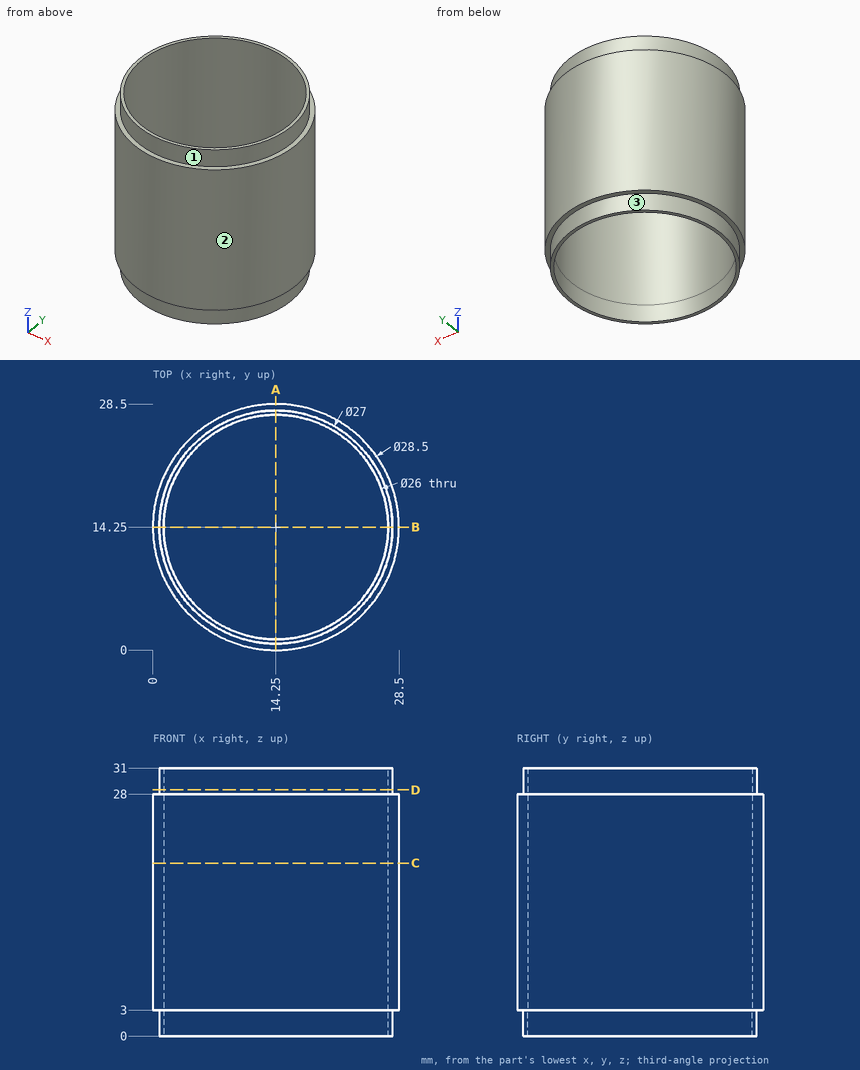
Design review of the part shown in the three views and the two pictorial views. Dimensions are in mm from the part's minimum x, y and z. A direction names the side the tool comes from. Round coordinates to 2 decimals unless told otherwise and drop trailing zeros. Order: outer loops, then holes, each group sorted by start corner. A loop starts at its lowest first (then second) coordinate and runs counter-clockwise, first axis right, second up. Notation, with made-up numbers: (-33.5, 32.25) - (-15.5, 32.25) arc R25 cw to (-15.5, 59.25) - close; hole circle Ø7 at (-40, 89). An arc over 180 degrees is marked (long way). Answer in a Markdown table with one row per item.
(1) Take a section at A-A on x = 14.25. Write out the cut boundary in (y, z).
Result set:
| item | result |
|---|---|
| outline | (0, 3) - (0.75, 3) - (0.75, 0) - (1.25, 0) - (1.25, 31) - (0.75, 31) - (0.75, 28) - (0, 28) - close; (27.25, 0) - (27.75, 0) - (27.75, 3) - (28.5, 3) - (28.5, 28) - (27.75, 28) - (27.75, 31) - (27.25, 31) - close |
(2) Take a section at D-D on z = 28.5. Write out the cut boundary in (x, y).
Result set:
| item | result |
|---|---|
| outline | circle Ø27 at (14.25, 14.25); hole circle Ø26 at (14.25, 14.25) |
(3) Clearance check with flat-ended pins moving along their axes: P1, Ø4, axis at x = 24.5, y = 3.5, coming from the -Z side; P2, Ø8, axis at x = 20.5, z = 26, coming from the +Y side; P3, Ø12, axis at y = 5, z = 16.5, coming from the +X side; P4, Ø8, axis at x = 7, y = 12.5, coming from the -Z side. State where each tip first meets the part, or that it passes through.
Result set:
| item | result |
|---|---|
| P1 | stops at z = 0 |
| P2 | stops at y = 28.32 |
| P3 | stops at x = 28.12 |
| P4 | passes through |
(4) Machinability: for the marked faces 1, 2 and 3, which of the approach directions +Z, -Z, +X, -X, +Y, -Y give a long, thin tool a straight path to every point of the face, cutting with its end or side? Answer none if there is none.
Result set:
| item | result |
|---|---|
| face 1 | +Z |
| face 2 | +Z, -Z |
| face 3 | -Z |
(5) For line 1 (Y direction, x = 14.25, z = 1.35); line 2 (X direction, y = 14, z = 27); line 3 (Y direction, x = 9, z = 12), list the stretches that pass through material, from the lowest coordinate up. Write a range as from..to.
Result set:
| item | result |
|---|---|
| line 1 | y = 0.75..1.25, 27.25..27.75 |
| line 2 | x = 0..1.25, 27.25..28.5 |
| line 3 | y = 1..2.36, 26.14..27.5 |
(6) Take a section at C-C on z = 20. Write out the cut boundary in (x, y).
Result set:
| item | result |
|---|---|
| outline | circle Ø28.5 at (14.25, 14.25); hole circle Ø26 at (14.25, 14.25) |
